Geometry check sheet. Reference: the model listing, model coordinates, mm. Face numbers are marked on the shaded views. A direction names the side the tool comes from. Coordinates: 2 decimals unless noted, no trailing zeros. Loops run counter-clockwise (first coordinate to the right, second up) from the corner with the lowest first, then second, coordinate; pieces in that order, holes last.
from build123d import *

# Parameters (mm, degrees)
CUT_EXTRUDE_1_DEPTH      = 18.592612086
CUT_EXTRUDE_1_DEPTH_BACK = 18.592612086
SKETCH_2_R               = 2


with BuildPart() as part:
    # 草图1 → 旋转1 (revolve)
    with BuildSketch(Plane.XY, mode=Mode.PRIVATE) as revolve_1_sk:
        with BuildLine():
            Line((6.5, 11), (6.5, 15))
            Line((6.5, 15), (4, 15))
            Line((4, 15), (4, 11.8))
            Line((4, 11.8), (0, 11.8))
            Line((0, 11.8), (0, 10.3))
            Line((0, 10.3), (3, 10.3))
            Line((3, 10.3), (3, 0))
            Line((3, 0), (5, 0))
            Line((5, 0), (5, 10))
            ThreePointArc((5, 10), (5.292893219, 10.707106781), (6, 11))
            Line((6, 11), (6.5, 11))
        make_face()
    revolve(revolve_1_sk.sketch.rotate(Axis((0, 11.8, 0), (0, -1, 0)), 180), axis=Axis((0, 11.8, 0), (0, -1, 0)))

    # 草图2 → 切除-拉伸1 (cut, two sides: drawn at the far end of the back side and taken through both)
    with BuildSketch(Plane.XY.offset(-CUT_EXTRUDE_1_DEPTH_BACK)):
        with Locations((0, 5)):
            Circle(SKETCH_2_R)
    extrude(amount=CUT_EXTRUDE_1_DEPTH + CUT_EXTRUDE_1_DEPTH_BACK, mode=Mode.SUBTRACT)


solid = part.part
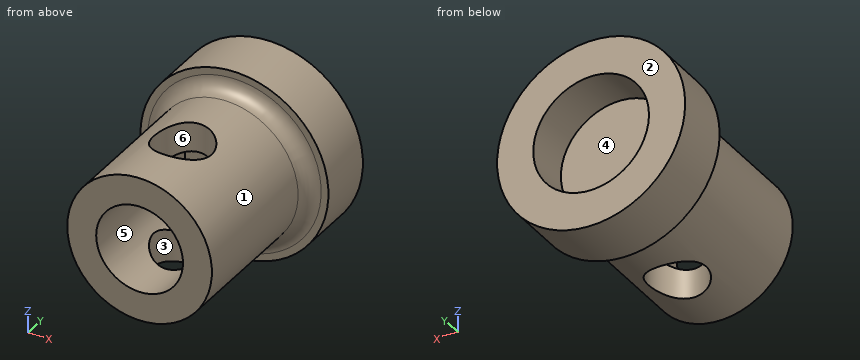
1) Section check C-C on z = 0. Record the cut outline in (x, y), and give its area (3 significant figures).
Data:
outline: (-6.5, 11) - (-6, 11) arc R1 cw to (-5, 10) - (-5, 0) - (-3, 0) - (-3, 10.3) - (3, 10.3) - (3, 0) - (5, 0) - (5, 10) arc R1 cw to (6, 11) - (6.5, 11) - (6.5, 15) - (4, 15) - (4, 11.8) - (-4, 11.8) - (-4, 15) - (-6.5, 15) - close
area: 75.0 mm2
2) Section check D-D on y = 14. Record the cut outline in (x, z).
Data:
outline: circle Ø13 at (0, 0); hole circle Ø8 at (0, 0)
3) Section check A-A on x = 0. Record the cut outline in (y, z), and give its area (3 significant figures).
Data:
outline: (0, -5) - (3, -5) - (3, -3) - (0, -3) - close; (0, 3) - (3, 3) - (3, 5) - (0, 5) - close; (7, -5) - (10, -5) arc R1 cw to (11, -6) - (11, -6.5) - (15, -6.5) - (15, -4) - (11.8, -4) - (11.8, 4) - (15, 4) - (15, 6.5) - (11, 6.5) - (11, 6) arc R1 cw to (10, 5) - (7, 5) - (7, 3) - (10.3, 3) - (10.3, -3) - (7, -3) - close
area: 59.0 mm2
4) Material ranges on probe 1 along Y at (x, z) = (0, -3.15); probe 2 along Z at (x, y) = (2, 7.5); probe 3 along X at (y, z) = (12.5, 0.75), recorded low to high.
Data:
probe 1: y = 0 to 3, 7 to 11.8
probe 2: z = -4.58 to -2.24, 2.24 to 4.58
probe 3: x = -6.46 to -3.93, 3.93 to 6.46
5) Section check B-B on y = 5. Record the cut outline in (x, z).
Data:
outline: (-2, -4.58) - (-2, -2.24) arc R3 cw to (-2, 2.24) - (-2, 4.58) arc R5 ccw to start; (2, -4.58) arc R5 ccw to (2, 4.58) - (2, 2.24) arc R3 cw to (2, -2.24) - close
6) Mould release check, pull along X, two halves, no side actions. Record for the marked faces 1, 2 and 3: +X half, -X half, draft (parallel to the pull), parting line (faces both ways), or undercut.
Data:
face 1: parting line
face 2: draft
face 3: undercut
7) Depth check by flat-ended pin: pin 1 (6.5 mm diameter, centred on x = 0, y = 5, fed in from +Z); pin 2 (3 mm diameter, centred on y = 4.5, z = -4.5, fed in from +X); pin 3 (4 mm diameter, centred on x = -1.5, z = -0.5, fed in from +Y). Enter the tip coordinate at first touch or a pass-through.
Data:
pin 1: stops at z = 5
pin 2: stops at x = 4
pin 3: stops at y = 11.8
8) Access from +Z, -Z, +X, -X, +Y, -Y to the whole of each face (thin tool, end or side, straight path). Record for the marked faces 4, 5 and 6.
Data:
face 4: +Y
face 5: -Y
face 6: +Z, -Z
